Input: part model. Units: mm. Frame: model coordinates. Face numbers are marked on the shaded views. A direction names the side the tool comes from. Coordinates: 2 decimals unless noted, no trailing zeros. Loops run counter-clockwise (first coordinate to the right, second up) from the corner with the lowest first, then second, coordinate; pieces in that order, holes last. Notation, with made-up numbers: (72, -10.75) - (122, -10.75) arc R17 cw to (122, 14.25) - close; hole circle Ø8 at (-16, 7). An arc over 180 degrees is marked (long way). Use a Markdown table: item, result. Add a question column.
1. Ray query, L1, parallel to Z at x = -16.5, y = 14; L2, parallel to X at y = 14, z = -5.5; L3, parallel to X at y = 15, z = -6.25. Return the intervals inside material, ascending. Write a range as [from, to].
2. Section query B-B on x = 7. Return the cut outline in (y, z), then the cut area to 4 significant figures.
3. Draft query along Z for the marked faces 6, 7 and 8. Return one class per face: released by +Z, released by -Z, zero draft, split by the parting line, or undercut.
4. Access query for the marked faces 1, 2, 3, 4 and 5. Directions: +Z, -Z, +X, -X, +Y, -Y. A direction counts if a zero-diameter tool reaches every point of the face in a straight line with its end or side. Return the directions, or none.
5. Section query D-D on y = -12.5. Return the cut outline in (x, z).
6. Contact query for flat-ended pins moving along their axis: P1, Ø11, axis at x = -12.5, y = 8.5, coming from the -Z side; P2, Ø6, axis at x = -7, z = -3.5, coming from the +Y side; P3, Ø2, axis at x = -17, y = -7, coming from the +Z side. Output: stop coordinate, or through.
7. Section query C-C on z = 9.25. Return the cut outline in (x, y), then the cut area to 3 significant figures.
8. Section query A-A on y = 8.5. Return the cut outline in (x, z).
Autodesk Inventor part; units mm, degrees
ref_plane "YZ Plane" through (0, 0, 0) normal (1, 0, 0) x (0, 1, 0)
ref_plane "XZ Plane" through (0, 0, 0) normal (0, 1, 0) x (-1, 0, 0)
ref_plane "XY Plane" through (0, 0, 0) normal (0, 0, 1) x (1, 0, 0)
sketch "스케치1" plane through (0, 0, 0) normal (0, 0, 1) x (1, 0, 0)
  line L0 (22.0682, -17.448) -> (-22.0682, -17.448)
  line L1 (-22.0682, -17.448) -> (-22.0682, 17.448)
  line L2 (-22.0682, 17.448) -> (22.0682, 17.448)
  line L3 (22.0682, 17.448) -> (22.0682, -17.448)
  line L4 (22.0682, -17.448) -> (-22.0682, 17.448) construction
  line L5 (-22.0682, -17.448) -> (22.0682, 17.448) construction
  point P0 (0, 0)
extrude "돌출1" add sketch "스케치1" along normal blind 10
sketch "스케치2" plane through (0, 0, 10) normal (0, 0, 1) x (1, 0, 0)
  line L0 (22.0682, 17.448) -> (-22.0682, 17.448)
  line L1 (-22.0682, -17.448) -> (22.0682, -17.448)
  line L2 (0, 17.448) -> (22.0682, -17.448)
  line L3 (0, 17.448) -> (-22.0682, -17.448)
  point P0 (0, 0)
extrude "돌출2" add sketch "스케치2" along normal blind 10
sketch "스케치3" plane through (0, 0, 0) normal (0, 0, -1) x (-1, 0, 0)
  line L0 (0, 17.448) -> (22.0682, 17.448)
  line L1 (-22.0682, -17.448) -> (22.0682, -17.448)
  line L2 (0, 17.448) -> (-22.0682, -17.448)
  line L3 (0, 17.448) -> (22.0682, -17.448)
  line L4 (22.0682, 17.448) -> (22.0682, -17.448)
  line L5 (0, 17.448) -> (22.0682, -17.448)
  point P0 (0, 0)
extrude "돌출3" add sketch "스케치3" along normal blind 10 contours L3 L1 L2
chamfer "모따기1" distance 5 angle 45 1 edges at (22.0682, 17.448, 5)
chamfer "모따기2" distance 5 angle 45 1 edges at (-22.0682, 17.448, 5)
properties part number "240503_3Dsketch08"
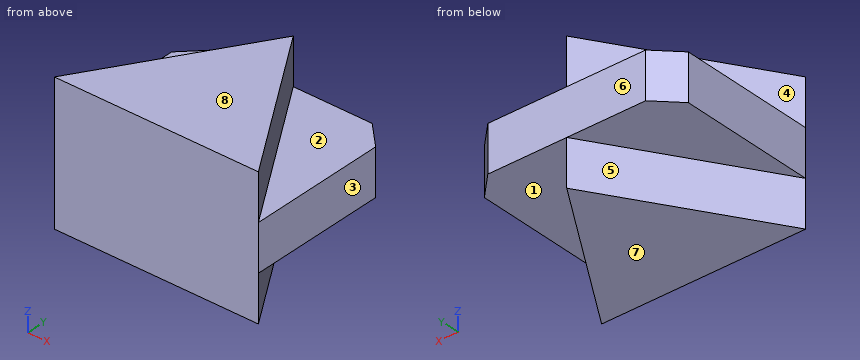
Resolved:
| question | item | result |
|---|---|---|
| 1 | L1 | [0, 10] |
| 1 | L2 | [-2.18, 2.18] |
| 1 | L3 | [-1.55, 1.55] |
| 2 | outline | (-17.45, -10) - (6.38, -10) - (6.38, 0) - (17.45, 0) - (17.45, 10) - (6.38, 10) - (6.38, 20) - (-17.45, 20) - close |
| 2 | area | 825.5 mm² |
| 3 | face 6 | zero draft |
| 3 | face 7 | released by -Z |
| 3 | face 8 | released by +Z |
| 4 | face 1 | -Z, +X, +Y |
| 4 | face 2 | +Z, +X, +Y |
| 4 | face 3 | +Z, -Z, +X, +Y, -Y |
| 4 | face 4 | +Z, -X, +Y |
| 4 | face 5 | -Z, -X, +Y |
| 5 | outline | (-22.07, 0) - (-18.94, 0) - (-18.94, -10) - (18.94, -10) - (18.94, 0) - (22.07, 0) - (22.07, 10) - (18.94, 10) - (18.94, 20) - (-18.94, 20) - (-18.94, 10) - (-22.07, 10) - close |
| 6 | P1 | z = 0 |
| 6 | P2 | y = 11.12 |
| 6 | P3 | z = 10 |
| 7 | outline | (-22.07, -17.45) - (22.07, -17.45) - (22.07, 12.45) - (17.07, 17.45) - (-17.07, 17.45) - (-22.07, 12.45) - close |
| 7 | area | 1,520 mm² |
| 8 | outline | (-22.07, 0) - (-5.66, 0) - (-5.66, -10) - (5.66, -10) - (5.66, 0) - (22.07, 0) - (22.07, 10) - (5.66, 10) - (5.66, 20) - (-5.66, 20) - (-5.66, 10) - (-22.07, 10) - close |
